from build123d import *

# Parameters (mm, degrees)
SKETCH1_R               = 10
BOSS_EXTRUDE1_DEPTH     = 60
CUT_EXTRUDE1_REACH      = 63.644
SKETCH2_R               = 3.75
CUT_EXTRUDE2_REACH      = 65.159
CUT_EXTRUDE2_END_RADIUS = 3.75
SKETCH3_R               = 1.25


with BuildPart() as part:
    # Sketch1 → Boss-Extrude1 (new body)
    with BuildSketch(Plane.XY):
        Circle(SKETCH1_R)
    extrude(amount=BOSS_EXTRUDE1_DEPTH)

    # Sketch2 → Cut-Extrude1 (cut, up to next)
    with BuildSketch(Plane(origin=(0, 0, 0), x_dir=(-1, 0, 0), z_dir=(0, 0, -1)), mode=Mode.PRIVATE) as cut_extrude1_sk1:
        Circle(SKETCH2_R)
    cut_extrude1_tool1 = extrude(cut_extrude1_sk1.sketch, amount=-CUT_EXTRUDE1_REACH, mode=Mode.PRIVATE) & part.part
    # Sketch2 → Cut-Extrude1 (cut, up to next)
    with BuildSketch(Plane(origin=(0, 0, 0), x_dir=(-1, 0, 0), z_dir=(0, 0, -1)), mode=Mode.PRIVATE) as cut_extrude1_sk2:
        with BuildLine():
            Line((-7.141428429, 7), (7.141428429, 7))
            ThreePointArc((7.141428429, 7), (0, 10), (-7.141428429, 7))
        make_face()
    cut_extrude1_tool2 = extrude(cut_extrude1_sk2.sketch, amount=-CUT_EXTRUDE1_REACH, mode=Mode.PRIVATE) & part.part
    add(cut_extrude1_tool1.solids().sort_by_distance((0, 0, 0))[0], mode=Mode.SUBTRACT)
    add(cut_extrude1_tool2.solids().sort_by_distance((0, 8.216904, 0))[0], mode=Mode.SUBTRACT)

    # Cut-Extrude2: up to this cylinder (the profile starts outside it)
    cut_extrude2_end = Plane(origin=(0, 0, 30), z_dir=(0, 0, -1)) * Cylinder(CUT_EXTRUDE2_END_RADIUS, 168.818, mode=Mode.PRIVATE)
    # Sketch3 → Cut-Extrude2 (cut, up to the surface)
    with BuildSketch(Plane(origin=(0, 7, 0), x_dir=(1, 0, 0), z_dir=(0, 1, 0)), mode=Mode.PRIVATE) as cut_extrude2_sk1:
        with Locations(Location((0, -15, 0), (0, 0, 270))):
            Circle(SKETCH3_R)
    cut_extrude2_tool1 = extrude(cut_extrude2_sk1.sketch, amount=-CUT_EXTRUDE2_REACH, mode=Mode.PRIVATE) - cut_extrude2_end
    add(cut_extrude2_tool1.solids().sort_by_distance((0, 7, 15))[0], mode=Mode.SUBTRACT)
    # Sketch3 → Cut-Extrude2 (cut, up to the surface)
    with BuildSketch(Plane(origin=(0, 7, 0), x_dir=(1, 0, 0), z_dir=(0, 1, 0)), mode=Mode.PRIVATE) as cut_extrude2_sk2:
        with Locations(Location((0, -45, 0), (0, 0, 270))):
            Circle(SKETCH3_R)
    cut_extrude2_tool2 = extrude(cut_extrude2_sk2.sketch, amount=-CUT_EXTRUDE2_REACH, mode=Mode.PRIVATE) - cut_extrude2_end
    add(cut_extrude2_tool2.solids().sort_by_distance((0, 7, 45))[0], mode=Mode.SUBTRACT)


solid = part.part
Input: part model. Units: mm. Frame: model coordinates. A direction names the side the tool comes from. Give positions to 0.01 mm unless a question says otherwise; leave off trailing zeros. Order: outer loops, then holes, each group sorted by start corner. A loop starts at its lowest first (then second) coordinate and runs counter-clockwise, first axis right, second up. Notation, with made-up numbers: (10.5, 43) - (40.5, 43) arc R17 cw to (40.5, 61) - close; hole circle Ø2 at (11.5, 54.25). An arc over 180 degrees is marked (long way). Answer as a JSON object with one key per item and string values. Group by question number.
Q1. Set-up query: faces 4 (the face through (0, 7, 30)), 5 (the face through (0.05, 5.29, 13.75)). Return all of +Z, -Z, +X, -X, +Y, -Y with unobstructed straight access to the full face (end or side cutting, diameter ignored); none if empty.
Q2. First-contact query: pin 1 Ø2 at (y, z) = (-7, 16.5) entering from -X; pin 2 Ø3 at (x, z) = (-2, 35) entering from -Y. Flat tips, straight axial feed; report the tip coordinate or a pass-through.
Q3. Line query: probe 1 along Z at (x, y) = (0, 6.1); probe 2 along X at (y, z) = (0.25, 4); probe 3 along X at (y, z) = (5, 15). Output: solid intervals per line, ascending.
Q4. Cut plane A-A, the plane y = 0. Output: boundary loops of the cut face in (x, z), then the cut area to 3 significant figures.
Q5. Mould query, pull axis X, two halves, no side actions, for faces 1 (the face through (2.1, -3.3, 0)), 2 (the face through (0, -10, 30)), 3 (the face through (0.05, 5.29, 43.75)). Classes: pulls with the +X half, pulls with the -X half, needs draft (parallel to the pull), parting line crosses it, or undercut.
Q6. Cut plane D-D, the plane z = 15. Output: boundary loops of the cut face in (x, y).
Q7. Cut plane B-B, the plane x = 0. Output: boundary loops of the cut face in (y, z), then the cut area to 3 significant figures.
Q8. Cut plane C-C, the plane x = 3. Output: boundary loops of the cut face in (y, z), then the cut area to 3 significant figures.
Results:
{
 "1": {"face 4": "+Z, -Z, +X, -X, +Y", "face 5": "+Y"},
 "2": {"pin 1": "x = -8", "pin 2": "y = -9.99"},
 "3": {"probe 1": "0 to 13.75, 16.25 to 43.75, 46.25 to 60", "probe 2": "-10 to -3.74, 3.74 to 10", "probe 3": "-8.66 to -1.25, 1.25 to 8.66"},
 "4": {"outline": "(-10, 0) - (-3.75, 0) - (-3.75, 60) - (-10, 60) - close; (3.75, 0) - (10, 0) - (10, 60) - (3.75, 60) - close", "area": "750 mm^2"},
 "5": {"face 1": "needs draft", "face 2": "parting line crosses it", "face 3": "undercut"},
 "6": {"outline": "(-7.14, 7) arc R10 ccw (long way) to (7.14, 7) - (1.25, 7) - (1.25, 3.54) arc R3.75 cw (long way) to (-1.25, 3.54) - (-1.25, 7) - close"},
 "7": {"outline": "(-10, 0) - (-3.75, 0) - (-3.75, 60) - (-10, 60) - close; (3.75, 0) - (7, 0) - (7, 13.75) - (3.75, 13.75) - close; (3.75, 16.25) - (7, 16.25) - (7, 43.75) - (3.75, 43.75) - close; (3.75, 46.25) - (7, 46.25) - (7, 60) - (3.75, 60) - close", "area": "554 mm^2"},
 "8": {"outline": "(-9.54, 0) - (-2.25, 0) - (-2.25, 60) - (-9.54, 60) - close; (2.25, 0) - (7, 0) - (7, 60) - (2.25, 60) - close", "area": "722 mm^2"}
}
